Check sheet for the modelled part. Datum: model origin and axes. Units: mm. A direction names the side the tool comes from. Give positions to 0.01 mm unless a question says otherwise; leave off trailing zeros. Order: outer loops, then holes, each group sorted by start corner. A loop starts at its lowest first (then second) coordinate and runs counter-clockwise, first axis right, second up.
```python
from build123d import *

# Parameters (mm, degrees)
SKETCH1_W           = 43
SKETCH1_H           = 43
SKETCH1_R           = 18.5
BOSS_EXTRUDE1_DEPTH = 5.5
SKETCH2_R           = 1.7
SKETCH2_R_2         = 2.5
BOSS_EXTRUDE2_DEPTH = 11
SKETCH3_R           = 1.7
CUT_EXTRUDE1_DEPTH  = 134.376282332
CUT_EXTRUDE11_DEPTH = 10
CUT_EXTRUDE12_DEPTH = 3
CUT_EXTRUDE13_DEPTH = 130.489381804


with BuildPart() as part:
    # Sketch1 → Boss-Extrude1 (new body)
    # profile 1 of 10: a face of its own
    with BuildSketch(Plane.XY):
        with BuildLine():
            Line((-33.5, -30), (-33.5, -4.850925931))
            ThreePointArc((-33.5, -4.850925931), (-34.593523061, -17.611516296), (-37.84220444, -30))
            Line((-37.84220444, -30), (-33.5, -30))
        make_face()
    # profile 2 of 10: a face of its own
    with BuildSketch(Plane.XY):
        Polygon((-21.5, -21.5), (-21.5, 21.5), (-33.5, 21.5), (-33.5, -4.850925931), (-33.5, -30), (0, -30), (33.5, -30), (33.5, -4.850925931), (33.5, 21.5), (21.5, 21.5), (21.5, -21.5), align=None)
    # profile 3 of 10: a face of its own
    with BuildSketch(Plane.XY):
        with BuildLine():
            ThreePointArc((37.84220444, -30), (34.593523061, -17.611516296), (33.5, -4.850925931))
            Line((33.5, -4.850925931), (33.5, -30))
            Line((33.5, -30), (37.84220444, -30))
        make_face()
    # profile 4 of 10: a face of its own
    with BuildSketch(Plane.XY):
        Rectangle(SKETCH1_W, SKETCH1_H)
        Circle(SKETCH1_R, mode=Mode.SUBTRACT)
    # profile 5 of 10: a face of its own
    with BuildSketch(Plane.XY):
        with BuildLine():
            Line((38.394173914, -31.5), (33.5, -31.5))
            Line((33.5, -31.5), (14.203872711, -31.5))
            ThreePointArc((14.203872711, -31.5), (34.722076366, -39.533108404), (51.594405594, -53.705335408))
            ThreePointArc((51.594405594, -53.705335408), (44.031058144, -43.175272448), (38.394173914, -31.5))
        make_face()
    # profile 6 of 10: a face of its own
    with BuildSketch(Plane.XY):
        with BuildLine():
            Line((-14.203872711, -31.5), (-33.5, -31.5))
            Line((-33.5, -31.5), (-38.394173914, -31.5))
            ThreePointArc((-38.394173914, -31.5), (-44.031058144, -43.175272448), (-51.594405594, -53.705335408))
            ThreePointArc((-51.594405594, -53.705335408), (-34.722076366, -39.533108404), (-14.203872711, -31.5))
        make_face()
    # profile 7 of 10: a face of its own
    with BuildSketch(Plane.XY):
        with BuildLine():
            Line((0, -30), (-33.5, -30))
            Line((-33.5, -30), (-33.5, -31.5))
            Line((-33.5, -31.5), (-14.203872711, -31.5))
            ThreePointArc((-14.203872711, -31.5), (-7.141428429, -30.376039749), (0, -30))
        make_face()
    # profile 8 of 10: a face of its own
    with BuildSketch(Plane.XY):
        with BuildLine():
            Line((33.5, -31.5), (33.5, -30))
            Line((33.5, -30), (0, -30))
            ThreePointArc((0, -30), (7.141428429, -30.376039749), (14.203872711, -31.5))
            Line((14.203872711, -31.5), (33.5, -31.5))
        make_face()
    # profile 9 of 10: a face of its own
    with BuildSketch(Plane.XY):
        with BuildLine():
            Line((37.84220444, -30), (33.5, -30))
            Line((33.5, -30), (33.5, -31.5))
            Line((33.5, -31.5), (38.394173914, -31.5))
            ThreePointArc((38.394173914, -31.5), (38.114193229, -30.751470427), (37.84220444, -30))
        make_face()
    # profile 10 of 10: a face of its own
    with BuildSketch(Plane.XY):
        with BuildLine():
            Line((-33.5, -31.5), (-33.5, -30))
            Line((-33.5, -30), (-37.84220444, -30))
            ThreePointArc((-37.84220444, -30), (-38.114193229, -30.751470427), (-38.394173914, -31.5))
            Line((-38.394173914, -31.5), (-33.5, -31.5))
        make_face()
    extrude(amount=BOSS_EXTRUDE1_DEPTH)

    # Sketch2 → Boss-Extrude2 (add)
    with BuildSketch(Plane.XY.offset(5.5)):
        with BuildLine():
            Line((-33.5, 30), (-33.5, 21.5))
            Line((-33.5, 21.5), (33.5, 21.5))
            Line((33.5, 21.5), (33.5, 30))
            ThreePointArc((33.5, 30), (35.66625593, 51.742394188), (39.542569928, 73.245848783))
            ThreePointArc((39.542569928, 73.245848783), (0, 122.5), (-39.542569928, 73.245848783))
            ThreePointArc((-39.542569928, 73.245848783), (-35.66625593, 51.742394188), (-33.5, 30))
        make_face()
        with Locations((-5.656854249, 76.343145751)):
            Circle(SKETCH2_R, mode=Mode.SUBTRACT)
        with Locations((5.656854249, 76.343145751)):
            Circle(SKETCH2_R, mode=Mode.SUBTRACT)
        with Locations((0, 82)):
            Circle(SKETCH2_R_2, mode=Mode.SUBTRACT)
        with Locations((-5.656854249, 87.656854249)):
            Circle(SKETCH2_R, mode=Mode.SUBTRACT)
        with Locations((5.656854249, 87.656854249)):
            Circle(SKETCH2_R, mode=Mode.SUBTRACT)
    extrude(amount=-BOSS_EXTRUDE2_DEPTH)

    # Sketch3 → Cut-Extrude1 (cut, through all)
    with BuildSketch(Plane.XY.offset(5.5)):
        with Locations((-15.5, 15.5)):
            Circle(SKETCH3_R)
        with Locations((15.5, 15.5)):
            Circle(SKETCH3_R)
        with Locations((15.5, -15.5)):
            Circle(SKETCH3_R)
        with Locations((-15.5, -15.5)):
            Circle(SKETCH3_R)
    extrude(amount=-CUT_EXTRUDE1_DEPTH, mode=Mode.SUBTRACT)

    # Sketch4 → Cut-Extrude11 (cut)
    with BuildSketch(Plane(origin=(0, 0, 0), x_dir=(-1, 0, 0), z_dir=(0, 0, -1))):
        with BuildLine():
            ThreePointArc((33.5, -18.5), (0, -24.278187239), (-33.5, -18.5))
            ThreePointArc((-33.5, -18.5), (-34.088098429, -18.288833154), (-34.674865885, -18.073995652))
            ThreePointArc((-34.674865885, -18.073995652), (-40.75024769, -37.021892063), (-51.594405594, -53.705335408))
            ThreePointArc((-51.594405594, -53.705335408), (0, -30), (51.594405594, -53.705335408))
            ThreePointArc((51.594405594, -53.705335408), (40.75024769, -37.021892063), (34.674865885, -18.073995652))
            ThreePointArc((34.674865885, -18.073995652), (34.088098429, -18.288833154), (33.5, -18.5))
        make_face()
    extrude(amount=-CUT_EXTRUDE11_DEPTH, mode=Mode.SUBTRACT)

    # Sketch5 → Cut-Extrude12 (cut)
    with BuildSketch(Plane.XY.offset(5.5)):
        Polygon((-7.331854249, 90.558039352), (-3.981854249, 90.558039352), (-2.306854249, 87.656854249), (-3.981854249, 84.755669147), (-7.331854249, 84.755669147), (-9.006854249, 87.656854249), align=None)
        Polygon((3.981854249, 90.558039352), (7.331854249, 90.558039352), (9.006854249, 87.656854249), (7.331854249, 84.755669147), (3.981854249, 84.755669147), (2.306854249, 87.656854249), align=None)
        Polygon((-7.331854249, 79.244330853), (-9.006854249, 76.343145751), (-7.331854249, 73.441960648), (-3.981854249, 73.441960648), (-2.306854249, 76.343145751), (-3.981854249, 79.244330853), align=None)
        Polygon((3.981854249, 79.244330853), (7.331854249, 79.244330853), (9.006854249, 76.343145751), (7.331854249, 73.441960648), (3.981854249, 73.441960648), (2.306854249, 76.343145751), align=None)
    extrude(amount=-CUT_EXTRUDE12_DEPTH, mode=Mode.SUBTRACT)

    # Sketch6 → Cut-Extrude13 (cut, through all)
    with BuildSketch(Plane(origin=(0, 0, -5.5), x_dir=(-1, 0, 0), z_dir=(0, 0, -1))):
        with BuildLine():
            Line((3.5, 46.5), (-3.5, 46.5))
            ThreePointArc((-3.5, 46.5), (-6.5, 49.5), (-3.5, 52.5))
            Line((-3.5, 52.5), (3.5, 52.5))
            ThreePointArc((3.5, 52.5), (6.5, 49.5), (3.5, 46.5))
        make_face()
    extrude(amount=-CUT_EXTRUDE13_DEPTH, mode=Mode.SUBTRACT)


solid = part.part
```
Q1. Sectioned sample at D-D, the plane y = -15.5. Record the cut outline in (x, z).
Q2. Sectioned sample at B-B, the plane z = -2.25. Record the cut outline in (x, y), plus the area to 3 significant figures.
Q3. Draft check along Y on faces 5 (the cylindrical face through (-14.7, 14, 2.8)), 6 (the flat face through (-1, 73, -5.5)). Enter one of: pulls with the +Y half, pulls with the -Y half, needs draft (parallel to the pull), parting line crosses it, or undercut.
Q4. Tool access check on faces 1 (the cylindrical face through (-6.5, 49.6, -0.1)), 2 (the flat face through (-4, 78, 2.5)), 3 (the flat face through (33.5, 16, 1)), 4 (the cylindrical face through (-35.71, 52.05, 0.08)). Record the directions out of +Z, -Z, +X, -X, +Y, -Y that give a thin tool (end or side, any length) a straight path to the whole face; none if there is none.
Q5. Sectioned sample at C-C, the plane x = -15.5. Record the cut outline in (y, z).
Q6. Go/stop test with flat-tipped pins: P1, Ø6, axis at y = 69.5, z = 1.5, coming from the -X side; P2, Ø3.5, axis at x = 5.5, z = 3.5, coming from the +Y side; P3, Ø3, axis at x = 19, z = -4, coming from the +Y side; P4, Ø3, axis at x = 5.66, y = 76.34, coming from the -Z side. Record where each tip stops, or that it passes through.
Q7. Material ranges on line 1 (Y direction, x = 0, z = 2.4); line 2 (Y direction, x = 15.5, z = 3.5); line 3 (X direction, y = 14.5, z = 4.75), recorded low to high.
Q8. Sectioned sample at A-A, the plane y = 0. Record the cut outline in (x, z).
Filled in:
1. outline: (-34.26, 0) - (-17.2, 0) - (-17.2, 5.5) - (-34.26, 5.5) - close; (-13.8, 0) - (-10.1, 0) - (-10.1, 5.5) - (-13.8, 5.5) - close; (10.1, 0) - (13.8, 0) - (13.8, 5.5) - (10.1, 5.5) - close; (17.2, 0) - (34.26, 0) - (34.26, 5.5) - (17.2, 5.5) - close
2. outline: (-39.54, 73.25) arc R276.5 cw to (-33.5, 30) - (-33.5, 21.5) - (33.5, 21.5) - (33.5, 30) arc R276.5 cw to (39.54, 73.25) arc R40.5 ccw (long way) to start; hole circle Ø3.4 at (-5.66, 76.34); hole circle Ø3.4 at (-5.66, 87.66); hole (-3.5, 46.5) - (3.5, 46.5) arc R3 ccw to (3.5, 52.5) - (-3.5, 52.5) arc R3 ccw to start; hole circle Ø5 at (0, 82); hole circle Ø3.4 at (5.66, 76.34); hole circle Ø3.4 at (5.66, 87.66)
2. area: 6,830 mm2
3. face 5: undercut
3. face 6: needs draft
4. face 1: +Z, -Z
4. face 2: +Z
4. face 3: +Z, -Z, +X
4. face 4: +Z, -Z, -X
5. outline: (-23.07, 0) - (-17.2, 0) - (-17.2, 5.5) - (-23.07, 5.5) - close; (-13.8, 0) - (-10.1, 0) - (-10.1, 5.5) - (-13.8, 5.5) - close; (10.1, 0) - (13.8, 0) - (13.8, 5.5) - (10.1, 5.5) - close; (17.2, 0) - (21.5, 0) - (21.5, -5.5) - (119.42, -5.5) - (119.42, 5.5) - (17.2, 5.5) - close
6. P1: stops at x = -39.38
6. P2: stops at y = 122.33
6. P3: stops at y = 118.52
6. P4: passes through
7. line 1: y = -24.28 to -18.5, 18.5 to 46.5, 52.5 to 79.5, 84.5 to 122.5
7. line 2: y = -23.07 to -17.2, -13.8 to -10.1, 10.1 to 13.8, 17.2 to 119.42
7. line 3: x = -33.5 to -16.87, -14.13 to -11.49, 11.49 to 14.13, 16.87 to 33.5
8. outline: (-33.5, 0) - (-18.5, 0) - (-18.5, 5.5) - (-33.5, 5.5) - close; (18.5, 0) - (33.5, 0) - (33.5, 5.5) - (18.5, 5.5) - close
